from build123d import *

# Parameters (mm, degrees)
F0_W     = 288.782075
F0_H     = 163.352266
F1_DEPTH = 5.08
F2_W     = 15.059188
F2_H     = 13.465754
F2_W_2   = 14.688864
F2_W_3   = 12.622907
F2_W_4   = 13.189614
F2_W_5   = 12.756806
F2_W_6   = 14.389988
F2_W_7   = 14.837095
F2_W_8   = 15.054709
F2_W_9   = 14.822775
F2_W_10  = 13.689365
F3_DEPTH = 5.842
F4_W     = 108.290506
F4_H     = 16.379602
F5_DEPTH = 5.842
F6_W     = 13.069794
F6_H     = 14.447321
F6_W_2   = 12.797505
F6_H_2   = 15.304588
F6_W_3   = 11.458419
F6_H_3   = 17.143417
F6_W_4   = 13.49812
F6_H_4   = 17.293982
F6_W_5   = 13.930906
F6_H_5   = 19.27505
F6_W_6   = 14.930427
F6_H_6   = 20.024683
F6_W_7   = 14.837095
F6_H_7   = 18.891268
F6_W_8   = 14.688871
F6_H_8   = 18.99891
F6_W_9   = 14.363708
F6_H_9   = 20.088118
F6_W_10  = 17.754339
F6_H_10  = 21.514323
F6_W_11  = 13.842166
F6_H_11  = 13.715633
F6_W_12  = 15.336946
F6_H_12  = 11.966504
F6_W_13  = 14.323011
F6_H_13  = 14.813163
F6_W_14  = 14.605261
F6_H_14  = 18.525428
F6_W_15  = 15.82228
F6_H_15  = 17.409948
F6_W_16  = 15.188619
F6_H_16  = 14.313415
F6_W_17  = 22.91315
F6_H_17  = 13.81641
F6_W_18  = 9.892102
F6_H_18  = 16.320752
F6_W_19  = 14.755823
F6_H_19  = 23.138981
F6_W_20  = 15.218579
F6_W_21  = 21.051738
F6_W_22  = 40.063784
F6_H_20  = 15.655063
F6_W_23  = 47.256365
F6_H_21  = 18.881655
F6_W_24  = 12.390971
F6_H_22  = 13.976591
F6_W_25  = 13.890229
F6_H_23  = 15.502113
F6_W_26  = 15.889235
F6_H_24  = 17.643357
F6_W_27  = 14.755819
F6_H_25  = 17.053898
F6_W_28  = 15.255572
F6_W_29  = 16.130783
F6_H_26  = 14.313408
F6_W_30  = 13.997871
F6_H_27  = 10.71711
F6_W_31  = 15.125354
F6_H_28  = 14.679253
F6_W_32  = 18.619925
F6_H_29  = 19.2571
F7_DEPTH = 6.858


with BuildPart() as f1:
    # F0 (on Top) → F1 (new body)
    with BuildSketch(Plane.XY):
        with Locations((-4.708923, 0.160061)):
            Rectangle(F0_W, F0_H)
    extrude(amount=F1_DEPTH)

    # F2 (on face) → F3 (join)
    with BuildSketch(Plane.XY.offset(5.08)):
        with Locations((-141.570367, 67.483317)):
            Rectangle(F2_W, F2_H)
        with Locations((-116.278112, 67.483317)):
            Rectangle(F2_W_2, F2_H)
        with Locations((-94.069093, 67.483317)):
            Rectangle(F2_W_3, F2_H)
        with Locations((-72.640784, 67.483317)):
            Rectangle(F2_W_4, F2_H)
        with Locations((-51.346382, 67.483317)):
            Rectangle(F2_W_5, F2_H)
        with Locations((-29.518751, 67.483317)):
            Rectangle(F2_W_6, F2_H)
        with Locations((-7.418547, 67.483317)):
            Rectangle(F2_W_7, F2_H)
        with Locations((15.999209, 67.483317)):
            Rectangle(F2_W_8, F2_H)
        with Locations((37.394049, 67.483317)):
            Rectangle(F2_W_9, F2_H)
        with Locations((58.271186, 67.483317)):
            Rectangle(F2_W_10, F2_H)
    extrude(amount=F3_DEPTH)

    # F4 (on face) → F5 (join)
    with BuildSketch(Plane.XY.offset(5.08)):
        with Locations((-36.067889, -73.326271)):
            Rectangle(F4_W, F4_H)
    extrude(amount=F5_DEPTH)

    # F6 (on face) → F7 (join)
    with BuildSketch(Plane.XY.offset(5.08)):
        with Locations((-142.565064, 41.434703)):
            Rectangle(F6_W, F6_H)
        with Locations((-117.223791, 41.863337)):
            Rectangle(F6_W_2, F6_H_2)
        with Locations((-94.610658, 42.782751)):
            Rectangle(F6_W_3, F6_H_3)
        with Locations((-72.486531, 43.047041)):
            Rectangle(F6_W_4, F6_H_4)
        with Locations((-50.759332, 44.011319)):
            Rectangle(F6_W_5, F6_H_5)
        with Locations((-29.248531, 43.244389)):
            Rectangle(F6_W_6, F6_H_6)
        with Locations((-7.418547, 41.669853)):
            Rectangle(F6_W_7, F6_H_7)
        with Locations((16.722579, 41.723674)):
            Rectangle(F6_W_8, F6_H_8)
        with Locations((37.164516, 42.268278)):
            Rectangle(F6_W_9, F6_H_9)
        with Locations((63.075055, 41.555175)):
            Rectangle(F6_W_10, F6_H_10)
        with Locations((-142.178878, 20.740474)):
            Rectangle(F6_W_11, F6_H_11)
        with Locations((-115.954071, 18.126391)):
            Rectangle(F6_W_12, F6_H_12)
        with Locations((-91.205612, 18.541897)):
            Rectangle(F6_W_13, F6_H_13)
        with Locations((-71.932961, 17.757031)):
            Rectangle(F6_W_14, F6_H_14)
        with Locations((-49.665319, 16.557304)):
            Rectangle(F6_W_15, F6_H_15)
        with Locations((-25.673699, 15.982273)):
            Rectangle(F6_W_16, F6_H_16)
        with Locations((-130.722303, -6.908205)):
            Rectangle(F6_W_17, F6_H_17)
        with Locations((-4.946051, 14.978605)):
            Rectangle(F6_W_18, F6_H_18)
        Polygon((7.496388, 23.138981), (0, 23.138981), (0, 6.818229), (-9.892102, 6.818229), (-9.892102, 0), (7.496388, 0), align=None)
        with Locations((21.294507, 11.56949)):
            Rectangle(F6_W_19, F6_H_19)
        with Locations((44.773805, 11.56949)):
            Rectangle(F6_W_20, F6_H_19)
        with Locations((69.993904, 11.56949)):
            Rectangle(F6_W_21, F6_H_19)
        with Locations((105.833657, 30.966513)):
            Rectangle(F6_W_22, F6_H_20)
        with Locations((110.443867, -17.380646)):
            Rectangle(F6_W_23, F6_H_21)
        with Locations((-105.748556, -6.988295)):
            Rectangle(F6_W_24, F6_H_22)
        with Locations((-87.151367, -7.751056)):
            Rectangle(F6_W_25, F6_H_23)
        with Locations((-67.871508, -8.821678)):
            Rectangle(F6_W_26, F6_H_24)
        with Locations((-46.293752, -8.526949)):
            Rectangle(F6_W_27, F6_H_25)
        with Locations((-24.733937, -8.526949)):
            Rectangle(F6_W_28, F6_H_25)
        with Locations((-1.82671, -16.142811)):
            Rectangle(F6_W_29, F6_H_26)
        with Locations((20.91553, -13.505332)):
            Rectangle(F6_W_30, F6_H_27)
        with Locations((44.727193, -14.763038)):
            Rectangle(F6_W_31, F6_H_28)
        with Locations((68.421774, -18.559552)):
            Rectangle(F6_W_32, F6_H_29)
    extrude(amount=F7_DEPTH)


solid = f1.part
Model file for the job. Use its own axes, mm. A direction names the side the tool comes from. Coordinates: 2 decimals unless noted, no trailing zeros. Loops run counter-clockwise (first coordinate to the right, second up) from the corner with the lowest first, then second, coordinate; pieces in that order, holes last. Notation, with made-up numbers: (52.5, -9) -> (89.5, -9) arc R16 cw to (89.5, -3) -> close; hole circle Ø3 at (14.5, -39). An arc over 180 degrees is marked (long way). Use one line per item in the form item = value. Start each with the question number.
(1) Cut at B-B on z = 7.25. Give the number of separate pieces and of enclosed holes in the cut face, and give its area (3 significant figures).
(2) Tool access for faces 4 (the flat face through (21, 0, 8)), 5 (the flat face through (-72, 27.02, 8)), 6 (the flat face through (-14.837, 67, 8)), 7 (the flat face through (-94.096, -8, 8)), 8 (the flat face through (-91, 11.135, 8)): list every direction of +Z, -Z, +X, -X, +Y, -Y with a clear straight run to the whole face (end or side of a thin tool).
(3) Probe probe 1 along Y at (x, z) = (65, 9); probe 2 along Y at (x, z) = (-90, 10); probe 3 along Y at (x, z) = (-111, 11.5). List the from-to ranges inside material, lowest first. Write a range as from..to.
(4) Flat gauge pins, fed straight in: pin 1 (5.5 mm diameter, centred on x = 68, z = 7.5, fed in from -Y); pin 2 (3.5 mm diameter, centred on y = -19, z = 10, fed in from +X); pin 3 (10 mm diameter, centred on x = -108, y = -63, fed in from +Z); pin 4 (5.5 mm diameter, centred on x = 19, z = 9.5, fed in from +Y). Where does each tip first touch, or does it go through?
(5) Cut at A-A on x = 90. Give the cut face in (y, z), and give its area (3 significant figures).
(6) Pull direction Y, two halves, no side cores. Call faces 1 (the flat face through (80.52, 11, 8)), 2 (the flat face through (44.346, 42, 8)), 3 (the flat face through (45, -22.103, 8)): pulls with the +Y half, pulls with the -Y half, needs draft (parallel to the pull), parting line crosses it, or undercut.
(7) Cut at C-C on y = -44.5. Give the cut face in (x, z), and give its area (3 significant figures).
Values:
q1.separate_pieces = 43
q1.enclosed_holes = 0
q1.area = 13,200 mm2
q2.face_4 = +Z, +X
q2.face_5 = +Z
q2.face_6 = +Z, +Y
q2.face_7 = +Z, -Y
q2.face_8 = +Z, -X
q3.probe_1 = -28.19..-8.93, 0..23.14, 30.8..52.31, 60.75..74.22
q3.probe_2 = -81.52..-65.14, -15.5..0, 11.14..25.95, 34.21..51.35, 60.75..74.22
q3.probe_3 = -13.98..0, 12.14..24.11, 34.21..49.52
q4.pin_1 = -81.52
q4.pin_2 = 134.07
q4.pin_3 = 5.08
q4.pin_4 = 74.22
q5.outline = (-81.52, 0) -> (81.84, 0) -> (81.84, 5.08) -> (38.79, 5.08) -> (38.79, 11.94) -> (23.14, 11.94) -> (23.14, 5.08) -> (-7.94, 5.08) -> (-7.94, 11.94) -> (-26.82, 11.94) -> (-26.82, 5.08) -> (-81.52, 5.08) -> close
q5.area = 1,070 mm2
q6.face_1 = needs draft
q6.face_2 = undercut
q6.face_3 = pulls with the -Y half
q7.outline = (-149.1, 0) -> (139.68, 0) -> (139.68, 5.08) -> (-149.1, 5.08) -> close
q7.area = 1,470 mm2
